The drawing under review shows one solid part. Ordinate dimensions are in mm from its lowest x, y, z. Coordinates: 2 decimals unless noted, no trailing zeros. Order: outer loops, then holes, each group sorted by start corner. A loop starts at its lowest first (then second) coordinate and runs counter-clockwise, first axis right, second up. Notation, with made-up numbers: M 60,66 L 78,66 A27 ccw 78,91 Z; hole C -11.5,-11.75 d1. An arc over 180 degrees is marked long. Answer as a JSON object with one key per item and string values.
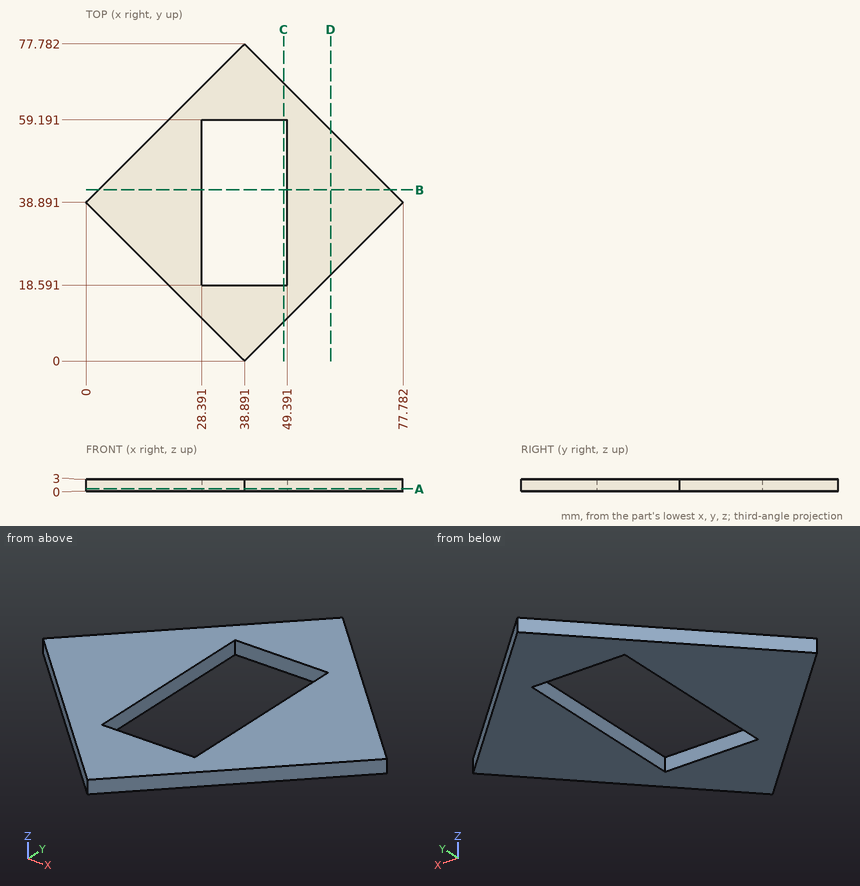
1) Add section D-D (x = 60). State the section outline as (y, z) points.
Taken from the geometry:
{"outline": "M 21.11,0 L 56.67,0 L 56.67,3 L 21.11,3 Z"}
2) Insertion check: pin 1 Ø0.9 at (x, z) = (36.5, 1.5) entering from +Y; pin 2 Ø1.5 at (x, z) = (54.5, 1.5) entering from -Y; pin 3 Ø1 at (x, z) = (21, 1.5) entering from +Y. Each pin has a flat end and moves straight along its axis. Give the tip position at first contact, or say it passes through.
Taken from the geometry:
{"pin 1": "stops at y = 75.84", "pin 2": "stops at y = 14.86", "pin 3": "stops at y = 60.39"}
3) Add section C-C (x = 48.5). State the section outline as (y, z) points.
Taken from the geometry:
{"outline": "M 9.61,0 L 18.59,0 L 18.59,3 L 9.61,3 Z; M 59.19,0 L 68.17,0 L 68.17,3 L 59.19,3 Z"}
4) Add section A-A (z = 0.6). State the section outline as (x, y) points.
Taken from the geometry:
{"outline": "M 0,38.89 L 38.89,0 L 77.78,38.89 L 38.89,77.78 Z; hole M 28.39,18.59 L 49.39,18.59 L 49.39,59.19 L 28.39,59.19 Z"}
5) Add section B-B (y = 42). State the section outline as (x, z) points.
Taken from the geometry:
{"outline": "M 3.11,0 L 28.39,0 L 28.39,3 L 3.11,3 Z; M 49.39,0 L 74.67,0 L 74.67,3 L 49.39,3 Z"}
6) To check wall thickness, follow L1, parallel to X at y = 49, z = 2.85; L2, parallel to X at y = 46, z = 2.75; L3, parallel to Y at x = 49, z = 0.6. State the ranges of each line that lie inside material, in increasing order.
Taken from the geometry:
{"L1": "x = 10.11 to 28.39, 49.39 to 67.67", "L2": "x = 7.11 to 28.39, 49.39 to 70.67", "L3": "y = 10.11 to 18.59, 59.19 to 67.67"}
